Geometry check sheet. Reference: the model listing, model coordinates, mm. A direction names the side the tool comes from. Give positions to 0.01 mm unless a question says otherwise; leave off trailing zeros. Loops run counter-clockwise (first coordinate to the right, second up) from the corner with the lowest first, then second, coordinate; pieces in that order, holes last. Notation, with made-up numbers: (6.5, 78.25) -> (10.5, 78.25) arc R6 cw to (10.5, 83.25) -> close; hole circle Ø11 at (66.25, -17.75). An arc over 180 degrees is marked (long way). One line per question, with ' | ' between items.
Autodesk Inventor part; units mm, degrees
ref_plane "YZ Plane" through (0, 0, 0) normal (1, 0, 0) x (0, 1, 0)
ref_plane "XZ Plane" through (0, 0, 0) normal (0, 1, 0) x (-1, 0, 0)
ref_plane "XY Plane" through (0, 0, 0) normal (0, 0, 1) x (1, 0, 0)
sketch "Sketch4" plane through (0, 0, 0) normal (1, 0, 0) x (0, 1, 0)
  circle A0 centre (0, 0) radius 7
  line L0 (4.899, 5) -> (-4.899, 5)
  line L1 (-4.899, -5) -> (4.899, -5)
  circle A1 centre (0, 0) radius 15
  circle A2 centre (0, 45) radius 2.5
  circle A3 centre (0, 45) radius 5
  line L2 (5, 45) -> (5, 22.3607)
  line L3 (-5, 45) -> (-5, 22.3607)
  line L4 (0, 0) -> (0, 45) construction
  arc A4 (5, 22.3607) -> (10, 11.1803) centre (20, 22.3607) ccw
  arc A5 (-10, 11.1803) -> (-5, 22.3607) centre (-20, 22.3607) ccw
  dimension "d29" = 30
  dimension "d18" = 14
  dimension "d19" = 10
  dimension "d30" = 10
  dimension "d31" = 5
  dimension "d33" = 45
extrude "Extrusion4" add sketch "Sketch4" along normal mid plane 5 contours L0 A0 | A0 L1 | A1
extrude "Extrusion5" add sketch "Sketch4" along normal mid plane 5 contours A1 A5 L3 A3 L2 A4 | A3
mirror "Mirror2" about plane through (0, 0, 0) normal (0, 0, 1) of "Extrusion5"
properties part number "panel" material "Aluminum 6061"
Item 1: Scan lines: probe 1 along Z at (x, y) = (1.35, 0); probe 2 along Y at (x, z) = (-1.1, -45); probe 3 along Z at (x, y) = (-1.1, -2). Record each from-to range of solid material in increasing order.
Result:
probe 1: -50 to -47.5, -42.5 to -5, 5 to 42.5, 47.5 to 50 | probe 2: -5 to -2.5, 2.5 to 5 | probe 3: -49.58 to -46.5, -43.5 to -5, 5 to 43.5, 46.5 to 49.58
Item 2: Sectioned sample at C-C (z = -35.5). Record the cut outline in (x, y).
Result:
outline: (-2.5, -5) -> (2.5, -5) -> (2.5, 5) -> (-2.5, 5) -> close
Item 3: Release check for a two-part mould opening along Y. For faces 6 (the face through (0, 7, 0)), 7 (the face through (-0.04, 6.34, 16.16)), 8 (the face through (0, -15, 0)), 9 (the face through (0, 0, 50)) record: pulls with the +Y half, pulls with the -Y half, needs draft (parallel to the pull), parting line crosses it, or undercut.
Result:
face 6: undercut | face 7: pulls with the +Y half | face 8: pulls with the -Y half | face 9: parting line crosses it
Item 4: Sectioned sample at B-B (x = 1.5). Record the cut outline in (y, z), plus the area to 3 significant figures.
Result:
outline: (-10, -11.18) arc R15 cw to (-5, -22.36) -> (-5, -45) arc R5 ccw to (5, -45) -> (5, -22.36) arc R15 cw to (10, -11.18) arc R15 ccw to (10, 11.18) arc R15 cw to (5, 22.36) -> (5, 45) arc R5 ccw to (-5, 45) -> (-5, 22.36) arc R15 cw to (-10, 11.18) arc R15 ccw to start; hole (-4.9, -5) -> (4.9, -5) arc R7 ccw to (4.9, 5) -> (-4.9, 5) arc R7 ccw to start; hole circle Ø5 at (0, -45); hole circle Ø5 at (0, 45) | area: 1,260 mm2
Item 5: Sectioned sample at D-D (y = 9). Record the cut outline in (x, z), plus the area to 3 significant figures.
Result:
outline: (-2.5, -12.16) -> (2.5, -12.16) -> (2.5, 12.16) -> (-2.5, 12.16) -> close | area: 122 mm2
Item 6: Set-up check for faces 1 (the face through (0, -7, 0)), 2 (the face through (0, 5, 34)), 3 (the face through (0, 5, -34)), 4 (the face through (0, -5, 34)), 5 (the face through (0, -5, -34)): record each of +Z, -Z, +X, -X, +Y, -Y from which the full face is reachable in a straight line by a thin tool's end or side.
Result:
face 1: +X, -X | face 2: +Z, +X, -X, +Y | face 3: -Z, +X, -X, +Y | face 4: +Z, +X, -X, -Y | face 5: -Z, +X, -X, -Y
Item 7: Depth check by flat-ended pin: pin 1 Ø1.5 at (x, z) = (0.5, -34) entering from +Y; pin 2 Ø3 at (x, y) = (1, 4) entering from -Z; pin 3 Ø2.5 at (x, y) = (1, 1) entering from -Z; pin 4 Ø1.5 at (x, z) = (1, 30.5) entering from -Y. Enter the tip coordinate at first touch or a pass-through.
Result:
pin 1: y = 5 | pin 2: z = -49.33 | pin 3: z = -50 | pin 4: y = -5
Item 8: Sectioned sample at A-A (y = 0). Record the cut outline in (x, z).
Result:
outline: (-2.5, -50) -> (2.5, -50) -> (2.5, -47.5) -> (-2.5, -47.5) -> close; (-2.5, -42.5) -> (2.5, -42.5) -> (2.5, -5) -> (-2.5, -5) -> close; (-2.5, 5) -> (2.5, 5) -> (2.5, 42.5) -> (-2.5, 42.5) -> close; (-2.5, 47.5) -> (2.5, 47.5) -> (2.5, 50) -> (-2.5, 50) -> close
